The model under review builds one solid part; all positions refer to its coordinate system, in mm. Face numbers are marked on the shaded views. A direction names the side the tool comes from. Round coordinates to 2 decimals unless told otherwise and drop trailing zeros. Write each loop counter-clockwise with the first axis right and the second up, starting at its lowest first coordinate (ties: lowest second). Pieces come first, ordered by that corner, then holes. Notation, with made-up numbers: (89.25, 47.25) -> (134.25, 47.25) arc R11 cw to (134.25, 51.25) -> close; hole circle Ø9 at (-26.75, 10). An arc over 180 degrees is marked (long way). Return JSON: item names as keys, results as strings. Group by question number.
1. Take a section at C-C, the plane y = 4. Write out the cut boundary in (x, z).
2. Take a section at B-B, the plane y = 11. Write out the cut boundary in (x, z).
3. Clearance check with flat-ended pins moving along their axes: P1, Ø6.5, axis at x = 118.12, z = 0, coming from the -Y side; P2, Ø3, axis at y = 0.5, z = -1.5, coming from the +X side; P3, Ø4, axis at y = 6, z = 1, coming from the -X side. State where each tip first meets the part, or that it passes through.
4. Tool access review of the marked faces 1, 2 and 3: name each direction out of +Z, -Z, +X, -X, +Y, -Y from which nothing blocks a thin tool from reaching the whole face with its end or side.
5. Take a section at A-A, the plane z = 0. Write out the cut boundary in (x, y), then the cut area to 3 significant figures.
6. For line 1 along Z through (x, y) = (6.35, 1.5); line 2 along Y through (x, z) = (85.5, -0.25); line 3 along Y through (x, z) = (17.5, 1.25), list the stretches that pass through material, from the lowest coordinate up. Write a range as from..to.
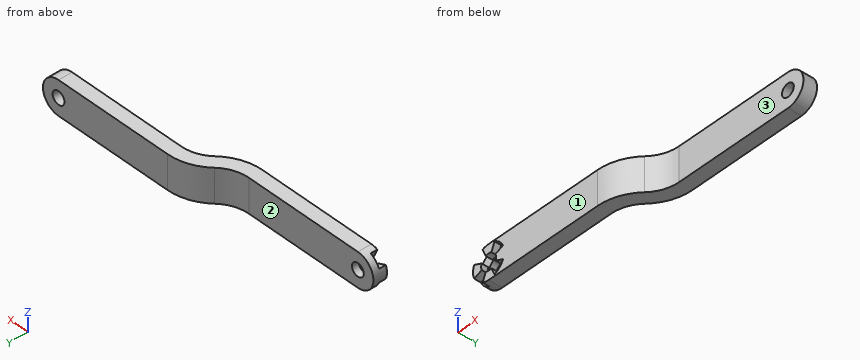
from build123d import *

# Parameters (mm, degrees)
SKETCH1_W               = 12.7
SKETCH1_H               = 5.08
CUT_EXTRUDE1_DEPTH      = 125.989350007
CUT_EXTRUDE1_DEPTH_BACK = 125.989350007
SKETCH5_R               = 2.413
FILLET1_RADIUS          = 6.35
FILLET1_LENGTH          = 5.08
FILLET2_RADIUS          = 6.35
FILLET2_LENGTH          = 5.08
CUT_EXTRUDE3_START      = -2.54
SKETCH6_R               = 2.413
CUT_EXTRUDE3_DEPTH      = 2.54


with BuildPart() as part:
    # Sweep1: sweep along a path in Sketch3
    with BuildLine(Plane.XY) as sweep1_path:
        Line((0, 0), (50.8, 0))
        ThreePointArc((50.8, 0), (56.988045526, 1.230878785), (62.234017215, 4.736125003))
        ThreePointArc((62.234017215, 4.736125003), (67.479988905, 8.241371221), (73.66803443, 9.472250006))
        Line((73.66803443, 9.472250006), (124.46803443, 9.472250006))
    # Sketch1 → Sweep1 (sweep)
    with BuildSketch(Plane(origin=(0, 0, 0), x_dir=(0, 0, -1), z_dir=(1, 0, 0))):
        Rectangle(SKETCH1_W, SKETCH1_H)
    sweep(path=sweep1_path.line)

    # Sketch5 → Cut-Extrude1 (cut, two sides: drawn at the far end of the back side and taken through both)
    with BuildSketch(Plane(origin=(0, 2.54, 0), x_dir=(1, 0, 0), z_dir=(0, 1, 0)).offset(-CUT_EXTRUDE1_DEPTH_BACK)):
        with Locations(Location((6.35, 0, 0), (0, 0, 270))):
            Circle(SKETCH5_R)
        with Locations(Location((118.11803443, 0, 0), (0, 0, 270))):
            Circle(SKETCH5_R)
    extrude(amount=CUT_EXTRUDE1_DEPTH + CUT_EXTRUDE1_DEPTH_BACK, mode=Mode.SUBTRACT)

    # Fillet1: full round fillet: the end face becomes a half cylinder, R = half its width
    fillet1_face = Plane((0, 0, 0), x_dir=(0, 1, 0), z_dir=(-1, 0, 0))  # on the end face: x along it, z out of the body
    fillet1_slab = fillet1_face.offset(-FILLET1_RADIUS / 2) * Box(FILLET1_LENGTH, 2 * FILLET1_RADIUS, FILLET1_RADIUS, mode=Mode.PRIVATE)  # the body's end, R deep
    fillet1_round = Plane((6.35, 0, 0), x_dir=(-1, 0, 0), z_dir=(0, 1, 0)) * Cylinder(FILLET1_RADIUS, FILLET1_LENGTH, mode=Mode.PRIVATE)  # its axis R under the face
    add(fillet1_slab - fillet1_round, mode=Mode.SUBTRACT)

    # Fillet2: full round fillet: the end face becomes a half cylinder, R = half its width
    fillet2_face = Plane((124.46803443, 9.472250006, 0), x_dir=(0, 1, 0), z_dir=(1, 0, 0))  # on the end face: x along it, z out of the body
    fillet2_slab = fillet2_face.offset(-FILLET2_RADIUS / 2) * Box(FILLET2_LENGTH, 2 * FILLET2_RADIUS, FILLET2_RADIUS, mode=Mode.PRIVATE)  # the body's end, R deep
    fillet2_round = Plane((118.11803443, 9.472250006, 0), x_dir=(1, 0, 0), z_dir=(0, 1, 0)) * Cylinder(FILLET2_RADIUS, FILLET2_LENGTH, mode=Mode.PRIVATE)  # its axis R under the face
    add(fillet2_slab - fillet2_round, mode=Mode.SUBTRACT)

    # Sketch6 → Cut-Extrude3 (cut)
    with BuildSketch(Plane.XZ.offset(2.54).offset(CUT_EXTRUDE3_START)):
        with BuildLine():
            Line((7.516419102, -2.815984815), (8.780039796, -5.866635031))
            ThreePointArc((8.780039796, -5.866635031), (10.840128061, -4.490128061), (12.216635031, -2.430039796))
            Line((12.216635031, -2.430039796), (9.165984815, -1.166419102))
            ThreePointArc((9.165984815, -1.166419102), (9.398, 0), (9.165984815, 1.166419102))
            Line((9.165984815, 1.166419102), (12.216635031, 2.430039796))
            ThreePointArc((12.216635031, 2.430039796), (10.840128061, 4.490128061), (8.780039796, 5.866635031))
            Line((8.780039796, 5.866635031), (7.516419102, 2.815984815))
            ThreePointArc((7.516419102, 2.815984815), (6.35, 3.048), (5.183580898, 2.815984815))
            Line((5.183580898, 2.815984815), (3.919960204, 5.866635031))
            ThreePointArc((3.919960204, 5.866635031), (1.859871939, 4.490128061), (0.483364969, 2.430039796))
            Line((0.483364969, 2.430039796), (3.534015185, 1.166419102))
            ThreePointArc((3.534015185, 1.166419102), (3.302, 0), (3.534015185, -1.166419102))
            Line((3.534015185, -1.166419102), (0.483364969, -2.430039796))
            ThreePointArc((0.483364969, -2.430039796), (1.859871939, -4.490128061), (3.919960204, -5.866635031))
            Line((3.919960204, -5.866635031), (5.183580898, -2.815984815))
            ThreePointArc((5.183580898, -2.815984815), (6.35, -3.048), (7.516419102, -2.815984815))
        make_face()
        with Locations(Location((6.35, 0, 0), (0, 0, 90))):
            Circle(SKETCH6_R, mode=Mode.SUBTRACT)
    extrude(amount=CUT_EXTRUDE3_DEPTH, mode=Mode.SUBTRACT)


solid = part.part
Output:
{
 "1": {"outline": "(56.94, -6.35) -> (65.22, -6.35) -> (65.22, 6.35) -> (56.94, 6.35) -> close"},
 "2": {"outline": "(67.6, -6.35) -> (118.12, -6.35) arc R6.35 ccw to (118.12, 6.35) -> (67.6, 6.35) -> close; hole circle Ø4.83 at (118.12, 0)"},
 "3": {"P1": "stops at y = 6.93", "P2": "stops at x = 63.02", "P3": "stops at x = 56.94"},
 "4": {"face 1": "+Z, -Z, +X, -X, -Y", "face 2": "+Z, -Z, -X, +Y", "face 3": "+Z, -Z, +X, -Y"},
 "5": {"outline": "(0, -2.54) -> (3.3, -2.54) -> (3.3, 0) -> (3.94, 0) -> (3.94, 2.54) -> (0, 2.54) -> close; (8.76, 0) -> (9.4, 0) -> (9.4, -2.54) -> (50.8, -2.54) arc R18.71 ccw to (64.03, 2.94) arc R13.63 cw to (73.67, 6.93) -> (115.71, 6.93) -> (115.71, 12.01) -> (73.67, 12.01) arc R18.71 ccw to (60.44, 6.53) arc R13.63 cw to (50.8, 2.54) -> (8.76, 2.54) -> close; (120.53, 6.93) -> (124.47, 6.93) -> (124.47, 12.01) -> (120.53, 12.01) -> close", "area": "593 mm^2"},
 "6": {"line 1": "z = -6.35..-2.41, 2.41..6.35", "line 2": "y = 6.93..12.01", "line 3": "y = -2.54..2.54"}
}
